```python
from build123d import *

# Parameters (mm, degrees)
SKIZZE1_R                       = 20
AUFSATZ_LINEAR_AUSTRAGEN1_DEPTH = 15
VERRUNDUNG1_R                   = 5
SKIZZE2_W                       = 10
SKIZZE2_H                       = 25
SCHNITT_LINEAR_AUSTRAGEN1_DEPTH = 10
SKIZZE3_R                       = 1.25
SCHNITT_LINEAR_AUSTRAGEN2_DEPTH = 5


with BuildPart() as part:
    # Skizze1 → Aufsatz-Linear austragen1 (new body)
    with BuildSketch(Plane.XY):
        Circle(SKIZZE1_R)
    extrude(amount=AUFSATZ_LINEAR_AUSTRAGEN1_DEPTH)

    # Verrundung1
    verrundung1_edges = [part.edges().sort_by_distance(p)[0] for p in [
        (-20, 0, 15),
    ]]
    fillet(verrundung1_edges, radius=VERRUNDUNG1_R)

    # Skizze2 → Schnitt-Linear austragen1 (cut)
    with BuildSketch(Plane(origin=(0, 0, 0), x_dir=(-1, 0, 0), z_dir=(0, 0, -1))):
        Rectangle(SKIZZE2_W, SKIZZE2_H)
    extrude(amount=-SCHNITT_LINEAR_AUSTRAGEN1_DEPTH, mode=Mode.SUBTRACT)

    # Skizze3 → Schnitt-Linear austragen2 (cut)
    with BuildSketch(Plane(origin=(0, 0, 0), x_dir=(-1, 0, 0), z_dir=(0, 0, -1))):
        with Locations((-13, 0)):
            Circle(SKIZZE3_R)
        with Locations((13, 0)):
            Circle(SKIZZE3_R)
    extrude(amount=-SCHNITT_LINEAR_AUSTRAGEN2_DEPTH, mode=Mode.SUBTRACT)


solid = part.part
```
The model under review builds one solid part; all positions refer to its coordinate system, in mm. A direction names the side the tool comes from. Round coordinates to 2 decimals unless told otherwise and drop trailing zeros. Loops run counter-clockwise (first coordinate to the right, second up) from the corner with the lowest first, then second, coordinate; pieces in that order, holes last. Notation, with made-up numbers: (20, -28) -> (61, -28) arc R14 ccw to (61, -3) -> close; hole circle Ø5 at (79, 50). An arc over 180 degrees is marked (long way). Answer as a JSON object with one key per item and string values. Group by question number.
1) We need section B-B on x = 0. Write out the cut boundary in (y, z), then the cut area to 3 significant figures.
2) For faces 1 (the face through (-5, 0, 5)), 2 (the face through (0, 0, 15)), list the 3-axis set-ups (+Z, -Z, +X, -X, +Y, -Y) from which the entire face can be reached by the end or side of a thin tool; tool diameter is ignored.
3) We need section D-D on z = 9.5. Write out the cut boundary in (x, y).
4) We need section A-A on z = 3. Write out the cut boundary in (x, y), then the cut area to 3 significant figures.
5) For pin 1 Ø1 at (y, z) = (4, 12.5) entering from +X; pin 2 Ø5 at (x, z) = (2, 5.5) entering from -Y; pin 3 Ø6 at (y, z) = (-14.5, 13.5) entering from +X, all flat-tipped, find the tip position at first contact; note any pin that passes through.
6) For line 1 (Z direction, x = -0.5, y = -6); line 2 (Y direction, x = 13, z = 4.25); line 3 (Y direction, x = -3.5, z = 6.5), list the stretches that pass through material, from the lowest coordinate up. Write a range as [from, to].
7) Mouldability with a two-part tool opening along Y and no side actions: class faces 3 (the face through (-4.336, -19.524, 4.93)), 4 (the face through (14.25, 0.05, 2.46)), 5 (the face through (9, 0, 0)) as released by +Y, released by -Y, zero draft, split by the parting line, or undercut.
8) We need section C-C on y = 0. Write out the cut boundary in (x, z), then the cut area to 3 significant figures.
Result set:
{
 "1": {"outline": "(-20, 0) -> (-12.5, 0) -> (-12.5, 10) -> (12.5, 10) -> (12.5, 0) -> (20, 0) -> (20, 10) arc R5 ccw to (15, 15) -> (-15, 15) arc R5 ccw to (-20, 10) -> close", "area": "339 mm²"},
 "2": {"face 1": "-Z", "face 2": "+Z, +X, -X, +Y, -Y"},
 "3": {"outline": "circle Ø40 at (0, 0); hole (-5, -12.5) -> (5, -12.5) -> (5, 12.5) -> (-5, 12.5) -> close"},
 "4": {"outline": "circle Ø40 at (0, 0); hole circle Ø2.5 at (-13, 0); hole (-5, -12.5) -> (5, -12.5) -> (5, 12.5) -> (-5, 12.5) -> close; hole circle Ø2.5 at (13, 0)", "area": "997 mm²"},
 "5": {"pin 1": "x = 19.19", "pin 2": "y = -20", "pin 3": "x = 15.56"},
 "6": {"line 1": "[10, 15]", "line 2": "[-15.2, -1.25], [1.25, 15.2]", "line 3": "[-19.69, -12.5], [12.5, 19.69]"},
 "7": {"face 3": "split by the parting line", "face 4": "undercut", "face 5": "zero draft"},
 "8": {"outline": "(-20, 0) -> (-14.25, 0) -> (-14.25, 5) -> (-11.75, 5) -> (-11.75, 0) -> (-5, 0) -> (-5, 10) -> (5, 10) -> (5, 0) -> (11.75, 0) -> (11.75, 5) -> (14.25, 5) -> (14.25, 0) -> (20, 0) -> (20, 10) arc R5 ccw to (15, 15) -> (-15, 15) arc R5 ccw to (-20, 10) -> close", "area": "464 mm²"}
}
